```python
from build123d import *

# Parameters (mm, degrees)
SKETCH1_R           = 40.4
SKETCH1_R_2         = 4.7625
BOSS_EXTRUDE1_DEPTH = 12.7
CUT_EXTRUDE1_DEPTH  = 5000
SKETCH3_R           = 4.7625
CUT_EXTRUDE2_DEPTH  = 5000
CUT_EXTRUDE3_DEPTH  = 20


with BuildPart() as part:
    # Sketch1 → Boss-Extrude1 (new body)
    with BuildSketch(Plane(origin=(0, 0, 0), x_dir=(1, 0, 0), z_dir=(0, 1, 0))):
        Polygon((205, 0), (305, 100), (305, 510), (205, 610), (-205, 610), (-305, 510), (-305, 100), (-205, 0), align=None)
        with Locations((-167.82128445, 168.589357775)):
            Circle(SKETCH1_R, mode=Mode.SUBTRACT)
        with Locations((-97, 168.589357775)):
            Circle(SKETCH1_R_2, mode=Mode.SUBTRACT)
        with Locations((97, 168.589357775)):
            Circle(SKETCH1_R_2, mode=Mode.SUBTRACT)
        with Locations((167.82128445, 168.589357775)):
            Circle(SKETCH1_R, mode=Mode.SUBTRACT)
        with Locations((-167.82128445, 441.410642225)):
            Circle(SKETCH1_R, mode=Mode.SUBTRACT)
        with Locations((-97, 441.410642225)):
            Circle(SKETCH1_R_2, mode=Mode.SUBTRACT)
        with Locations((97, 441.410642225)):
            Circle(SKETCH1_R_2, mode=Mode.SUBTRACT)
        with Locations((167.82128445, 441.410642225)):
            Circle(SKETCH1_R, mode=Mode.SUBTRACT)
    extrude(amount=BOSS_EXTRUDE1_DEPTH)

    # Sketch2 → Cut-Extrude1 (cut)
    with BuildSketch(Plane(origin=(0, 12.7, 0), x_dir=(1, 0, 0), z_dir=(0, 1, 0))):
        Polygon((-111, 69), (-180, 0), (180, 0), (111, 69), align=None)
    extrude(amount=-CUT_EXTRUDE1_DEPTH, mode=Mode.SUBTRACT)

    # Sketch3 → Cut-Extrude2 (cut)
    with BuildSketch(Plane(origin=(0, 12.7, 0), x_dir=(1, 0, 0), z_dir=(0, 1, 0))):
        with Locations((-205, 22.45771137)):
            Circle(SKETCH3_R)
        with Locations((205, 22.45771137)):
            Circle(SKETCH3_R)
        with Locations((-282.54228863, 100)):
            Circle(SKETCH3_R)
        with Locations((282.54228863, 100)):
            Circle(SKETCH3_R)
        with Locations((282.54228863, 510)):
            Circle(SKETCH3_R)
        with Locations((205, 587.54228863)):
            Circle(SKETCH3_R)
        with Locations((-205, 587.54228863)):
            Circle(SKETCH3_R)
        with Locations((-282.54228863, 510)):
            Circle(SKETCH3_R)
    extrude(amount=-CUT_EXTRUDE2_DEPTH, mode=Mode.SUBTRACT)

    # Sketch4 → Cut-Extrude3 (cut)
    with BuildSketch(Plane(origin=(0, 12.7, 0), x_dir=(1, 0, 0), z_dir=(0, 1, 0))):
        Polygon((-208.22128445, 360.529405268), (-97, 401.010642225), (-97, 208.989357775), (-208.22128445, 249.470594732), align=None)
        Polygon((208.22128445, 249.470594732), (208.22128445, 360.529405268), (97, 401.010642225), (97, 208.989357775), align=None)
    extrude(amount=-CUT_EXTRUDE3_DEPTH, mode=Mode.SUBTRACT)


solid = part.part
```
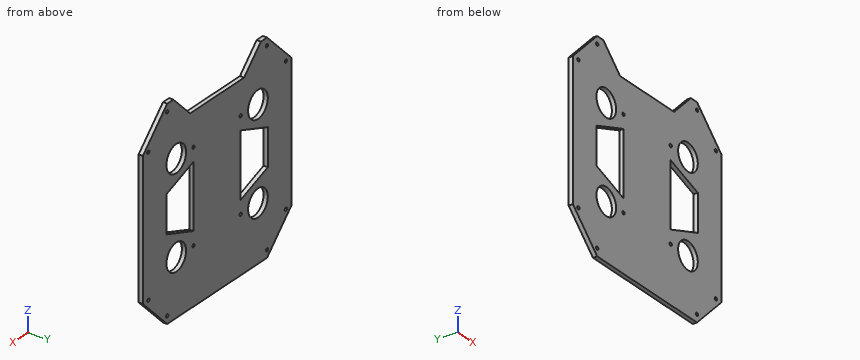
Design review of the part built by this model. Coordinates are the model's own, in mm. Give positions to 0.01 mm unless a question says otherwise; leave off trailing zeros. Write each loop counter-clockwise with the first axis right and the second up, starting at its lowest first coordinate (ties: lowest second). Pieces come first, ordered by that corner, then holes. Notation, with made-up numbers: (20, -19) - (46, -19) arc R21 ccw to (46, -9) - close; hole circle Ø1 at (10.5, -40). An arc over 180 degrees is marked (long way). Return JSON: item names as keys, results as strings. Group by question number.
(1) We need section C-C, the plane z = -555. Give the boundary of the cut face in (x, y).
(2) To check wall thickness, follow probe 1 along X at (y, z) = (7.5, -275.5); probe 2 along X at (y, z) = (7.5, -100); probe 3 along Z at (x, y) = (134.5, 3.75). State the ranges of each line that lie inside material, in increasing order.
(3) We need section A-A, the plane z = -304. Give the boundary of the cut face in (x, y), then the cut area to 3 significant figures.
(4) We need section D-D, the plane x = -228. Give the boundary of the cut face in (y, z).
(5) We need section B-B, the plane x = 147. Give the boundary of the cut face in (y, z).
Reported:
{
 "1": {"outline": "(-260, 0) - (260, 0) - (260, 12.7) - (-260, 12.7) - close"},
 "2": {"probe 1": "x = -305 to -208.22, -97 to 97, 208.22 to 305", "probe 2": "x = -305 to -287.3, -277.78 to 277.78, 287.3 to 305", "probe 3": "z = -610 to -464.25, -418.57 to -387.36, -222.64 to -191.43, -145.75 to -45.5"},
 "3": {"outline": "(-305, 0) - (-208.22, 0) - (-208.22, 12.7) - (-305, 12.7) - close; (-97, 0) - (97, 0) - (97, 12.7) - (-97, 12.7) - close; (208.22, 0) - (305, 0) - (305, 12.7) - (208.22, 12.7) - close", "area": "4,920 mm2"},
 "4": {"outline": "(0, -587) - (12.7, -587) - (12.7, -23) - (0, -23) - close"},
 "5": {"outline": "(0, -610) - (12.7, -610) - (12.7, -476.03) - (0, -476.03) - close; (0, -406.79) - (12.7, -406.79) - (12.7, -382.81) - (0, -382.81) - close; (0, -227.19) - (12.7, -227.19) - (12.7, -203.21) - (0, -203.21) - close; (0, -133.97) - (12.7, -133.97) - (12.7, -33) - (0, -33) - close"}
}
